Check sheet for the modelled part. Datum: model origin and axes. Units: mm. Face numbers are marked on the shaded views. A direction names the side the tool comes from. Round coordinates to 2 decimals unless told otherwise and drop trailing zeros. Write each loop counter-clockwise with the first axis right and the second up, starting at its lowest first coordinate (ties: lowest second). Pieces come first, ordered by that corner, then holes. Notation, with made-up numbers: (14.25, -28.75) -> (49.25, -28.75) arc R26 cw to (49.25, 2.25) -> close; hole circle Ø4 at (-34.75, 80.25). An arc over 180 degrees is marked (long way). Put each result on its own line as item: value. Start each with the question number.
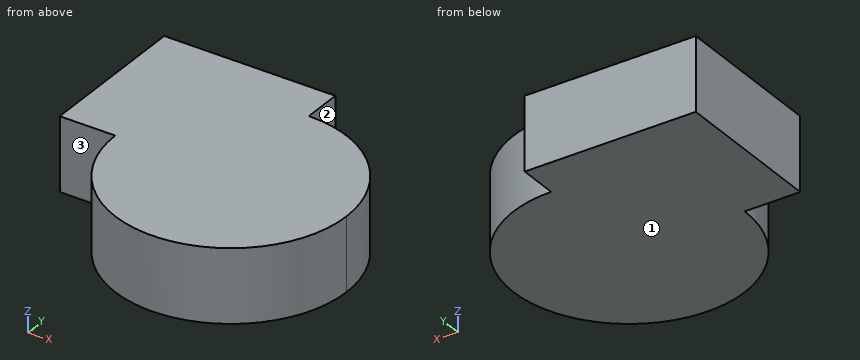
from build123d import *

# Parameters (mm, degrees)
F1_DEPTH = 25
F2_DEPTH = 25


with BuildPart() as f1:
    # F0 (on Top) → F1 (new body)
    with BuildSketch(Plane.XY):
        with BuildLine():
            ThreePointArc((-39.348634, 0), (-27.823686, 27.823686), (0, 39.348634))
            Line((0, 39.348634), (0, 52.689109))
            Line((0, 52.689109), (-58.225289, 52.689109))
            Line((-58.225289, 52.689109), (-58.225289, 0))
            Line((-58.225289, 0), (-39.348634, 0))
        make_face()
    extrude(amount=F1_DEPTH)

    # F0 (on Top) → F2 (join)
    with BuildSketch(Plane.XY):
        with BuildLine():
            ThreePointArc((-39.348634, 0), (0, -39.348634), (39.348634, 0))
            ThreePointArc((39.348634, 0), (27.823686, 27.823686), (0, 39.348634))
            Line((0, 39.348634), (0, 0))
            Line((0, 0), (-39.348634, 0))
        make_face()
        with BuildLine():
            Line((0, 0), (0, 39.348634))
            ThreePointArc((0, 39.348634), (-27.823686, 27.823686), (-39.348634, 0))
            Line((-39.348634, 0), (0, 0))
        make_face()
    extrude(amount=F2_DEPTH)


solid = f1.part
1. Section check B-B, the plane x = -50. Enter the section's corners in (y, z).
2. Gauge pin test, flat ends, axial feed: P1, Ø4, axis at y = -14.5, z = 20.5, coming from the +X side; P2, Ø1.5, axis at y = -23.5, z = 15.5, coming from the +X side; P3, Ø1.5, axis at x = -8, z = 19, coming from the -Y side. Record the tip position at first contact, or that the pin passes through.
3. Section check A-A, the plane z = 23. Enter the section's corners in (x, y).
4. Access from +Z, -Z, +X, -X, +Y, -Y to the whole of each face (thin tool, end or side, straight path). Record for the marked faces 1, 2 and 3.
5. Material ranges on L1, parallel to X at y = -1, z = 22.5; L2, parallel to X at y = 41, z = 10; L3, parallel to Y at x = -26, z = 17.5, recorded low to high. Write a range as [from, to].
6. Section check C-C, the plane y = 28. Enter the section's corners in (x, z).
Reply:
1. outline: (0, 0) -> (52.69, 0) -> (52.69, 25) -> (0, 25) -> close
2. P1: stops at x = 37.31
2. P2: stops at x = 32.11
2. P3: stops at y = -38.67
3. outline: (-58.23, 0) -> (-39.35, 0) arc R39.35 ccw (long way) to (0, 39.35) -> (0, 52.69) -> (-58.23, 52.69) -> close
4. face 1: -Z, +X, -X, +Y, -Y
4. face 2: +Z, -Z, +X, +Y
4. face 3: +Z, -Z, -X, -Y
5. L1: x = [-39.34, 39.34]
5. L2: x = [-58.23, 0]
5. L3: y = [-29.53, 52.69]
6. outline: (-58.23, 0) -> (27.65, 0) -> (27.65, 25) -> (-58.23, 25) -> close
